Part model, mm, in its own coordinate system. Give positions to 0.01 mm unless a question says otherwise; leave off trailing zeros. Order: outer loops, then holes, each group sorted by start corner. A loop starts at its lowest first (then second) coordinate and runs counter-clockwise, first axis right, second up. Notation, with made-up numbers: (61, -11) - (82, -11) arc R23 cw to (82, 24) - close; hole circle Ø6 at (37.5, 16). An arc over 180 degrees is marked (long way). One line per item, written item: value.
Autodesk Inventor part; units mm, degrees
ref_plane "YZ Plane" through (0, 0, 0) normal (1, 0, 0) x (0, 1, 0)
ref_plane "XZ Plane" through (0, 0, 0) normal (0, 1, 0) x (-1, 0, 0)
ref_plane "XY Plane" through (0, 0, 0) normal (0, 0, 1) x (1, 0, 0)
sketch "スケッチ1" plane through (0, 0, 0) normal (0, 0, 1) x (1, 0, 0)
  line L0 (0, 0) -> (9, 0)
  line L1 (9, 0) -> (9, -9)
  line L2 (9, -9) -> (0, -9)
  line L3 (0, -9) -> (0, 0)
  line L4 (1.2, -1.2) -> (7.8, -1.2)
  line L5 (7.8, -1.2) -> (7.8, -7.8)
  line L6 (7.8, -7.8) -> (1.2, -7.8)
  line L7 (1.2, -7.8) -> (1.2, -1.2)
  dimension "d0" = 9
  dimension "d1" = 9
  dimension "d2" = 6.6
  dimension "d3" = 6.6
  dimension "d4" = 1.2
  dimension "d5" = 1.2
extrude "押し出し1" add sketch "スケッチ1" along normal blind 80
sketch "スケッチ3" plane through (0, -9, 0) normal (0, -1, 0) x (1, 0, 0)
  line L0 (0, 80) -> (9, 80)
  line L1 (0, 0) -> (9, 0)
  line L2 (9, 0) -> (9, 80)
  point P0 (4.5, 4.5)
  point P1 (4.5, 75.5)
  dimension "d20" = 4.5
  dimension "d21" = 4.5
  dimension "d22" = 4.5
  dimension "d23" = 4.5
hole "穴2" at (4.5, -9, 4.5) at (4.5, -9, 75.5) direction (0, 1, 0) diameter 3 end through all
sketch "スケッチ4" plane through (9, -9, 0) normal (1, 0, 0) x (0, 0, -1)
  line L0 (0, 0) -> (0, 9)
  line L1 (-80, 0) -> (-80, 9)
  line L2 (0, 0) -> (-80, 0)
  point P0 (-13.5, 4.5)
  point P1 (-66.5, 4.5)
  dimension "d31" = 13.5
  dimension "d32" = 13.5
  dimension "d33" = 4.5
  dimension "d34" = 4.5
hole "穴3" at (9, -4.5, 13.5) at (9, -4.5, 66.5) direction (-1, 0, 0) diameter 3 end through all
sketch "スケッチ5" plane through (0, -9, 0) normal (0, -1, 0) x (1, 0, 0)
  line L0 (0, 0) -> (0, 80)
  line L1 (0, 0) -> (9, 0)
  point P0 (4.5, 20)
  dimension "d42" = 4.5
  dimension "d43" = 20
hole "穴4" at (4.5, -9, 20) direction (0, 1, 0) diameter 3 end through all
sketch "スケッチ6" plane through (0, -9, 0) normal (0, -1, 0) x (1, 0, 0)
  circle A0 centre (4.5, 4.5) radius 1.5
  circle A1 centre (4.5, 75.5) radius 1.5
  line L0 (4.5, 4.5) -> (4.5, 75.5)
  circle A2 centre (4.5, 20) radius 1.5
  point P0 (0, 0)
  point P1 (4.5, 12.25)
  point P2 (4.5, 26.1667)
  point P3 (4.5, 32.3333)
  point P4 (4.5, 38.5)
  point P5 (4.5, 44.6667)
  point P6 (4.5, 50.8333)
  point P7 (4.5, 57)
  point P8 (4.5, 63.1667)
  point P9 (4.5, 69.3333)
  dimension "d51" = 15.5
  dimension "d52" = 7.75
  dimension "d53" = 55.5
  dimension "d54" = 6.1667
  dimension "d57" = 6.1667
hole "穴5" at (4.5, -9, 12.25) at (4.5, -9, 26.1667) at (4.5, -9, 32.3333) at (4.5, -9, 38.5) at (4.5, -9, 44.6667) at (4.5, -9, 50.8333) at (4.5, -9, 57) at (4.5, -9, 63.1667) at (4.5, -9, 69.3333) direction (0, 1, 0) diameter 5 end through all
sketch "スケッチ7" plane through (0, -9, 0) normal (-1, 0, 0) x (0, 0, 1)
  circle A0 centre (66.5, 4.5) radius 1.5
  line L0 (80, 9) -> (80, 0)
  line L1 (0, 9) -> (80, 9)
  line L2 (0, 9) -> (0, 0)
  circle A1 centre (13.5, 4.5) radius 1.5
  circle A2 centre (66.5, 4.5) radius 1.5
  line L3 (13.5, 4.5) -> (66.5, 4.5)
  point P0 (6.75, 4.5)
  point P1 (73.25, 4.5)
  point P2 (20.125, 4.5)
  point P3 (26.75, 4.5)
  point P4 (33.375, 4.5)
  point P5 (40, 4.5)
  point P6 (46.625, 4.5)
  point P7 (53.25, 4.5)
  point P8 (59.875, 4.5)
  dimension "d69" = 6.75
  dimension "d70" = 13.5
  dimension "d71" = 4.5
  dimension "d72" = 6.75
  dimension "d73" = 4.5
  dimension "d74" = 53
  dimension "d75" = 6.625
  dimension "d78" = 6.625
hole "穴6" at (0, -4.5, 6.75) at (0, -4.5, 73.25) at (0, -4.5, 20.125) at (0, -4.5, 26.75) at (0, -4.5, 33.375) at (0, -4.5, 40) at (0, -4.5, 46.625) at (0, -4.5, 53.25) at (0, -4.5, 59.875) direction (1, 0, 0) diameter 5 end through all
properties part number "上下直動9x9_1_CPY" material "アルミニウム 6061"
1) Slice it at B-B on z = 40. Write the cut outline in (x, y).
Answer:
outline: (0, -9) - (2.5, -9) - (2.5, -7.8) - (1.2, -7.8) - (1.2, -7) - (0, -7) - close; (0, -2) - (1.2, -2) - (1.2, -1.2) - (2.5, -1.2) - (2.5, 0) - (0, 0) - close; (6.5, -9) - (9, -9) - (9, -7) - (7.8, -7) - (7.8, -7.8) - (6.5, -7.8) - close; (6.5, -1.2) - (7.8, -1.2) - (7.8, -2) - (9, -2) - (9, 0) - (6.5, 0) - close
2) Slice it at A-A on z = 6.75. Write the cut outline in (x, y).
Answer:
outline: (0, -9) - (9, -9) - (9, -7) - (7.8, -7) - (7.8, -7.8) - (1.2, -7.8) - (1.2, -7) - (0, -7) - close; (0, -2) - (1.2, -2) - (1.2, -1.2) - (7.8, -1.2) - (7.8, -2) - (9, -2) - (9, 0) - (0, 0) - close
3) Slice it at D-D on z = 20. Write the cut outline in (x, y).
Answer:
outline: (0, -9) - (3, -9) - (3, -7.8) - (1.2, -7.8) - (1.2, -7) - (0, -7) - close; (0, -2) - (1.2, -2) - (1.2, -1.2) - (3, -1.2) - (3, 0) - (0, 0) - close; (6, -9) - (9, -9) - (9, -7) - (7.8, -7) - (7.8, -7.8) - (6, -7.8) - close; (6, -1.2) - (7.8, -1.2) - (7.8, -2) - (9, -2) - (9, 0) - (6, 0) - close
4) Slice it at C-C on y = -4.5. Count the separate pieces of the cut face and the enclosed holes in it, then the cut area to 3 significant figures.
Answer:
separate pieces: 24
enclosed holes: 0
area: 69.6 mm2
5) Drop flat-ended pins along their axis: P1, Ø4, axis at x = 2.5, y = -6, coming from the -Z side; P2, Ø4, axis at x = 4.5, z = 69.33, coming from the -Y side. Give the stop position or say it passes through.
Answer:
P1: stops at z = 0
P2: passes through
6) Wall check: line 1 along X through (y, z) = (-1.75, 25); line 2 along Y through (x, z) = (7, 17); line 3 along Y through (x, z) = (8, 60). Give the ranges that are in metal, low to high. Write a range as [from, to].
Answer:
line 1: x = [0, 1.2], [7.8, 9]
line 2: y = [-9, -7.8], [-1.2, 0]
line 3: y = [-9, -7], [-2, 0]
7) Two-plate mould, pull along Z, no slides. Class faces 1 (the face through (9, -1, 39)), 2 (the face through (8.408, -4.61, 70.752)): pulls with the +Z half, pulls with the -Z half, needs draft (parallel to the pull), parting line crosses it, or undercut.
Answer:
face 1: needs draft
face 2: undercut
